For this review, take the finished solid that the model builds, in its own axes (mm). A direction names the side the tool comes from. Give positions to 0.01 mm unless a question says otherwise; leave off trailing zeros. Write each loop counter-clockwise with the first axis right and the second up, starting at its lowest first coordinate (ties: lowest second). Pieces come first, ordered by that corner, then holes.
Q1. We need section D-D (z = 2.5). Write out the cut boundary in (x, y), then the cut area to 3 significant figures.
Q2. For line 1 (Z direction, x = -2.5, y = 9.5); line 2 (Y direction, x = 0, z = 3.5); line 3 (Y direction, x = -16, z = 0.25), list the stretches that pass through material, from the lowest coordinate up.
Q3. We need section A-A (x = 16). Write out the cut boundary in (y, z) (3 decimals).
Q4. Machinability: for faces 4 (the flat face through (-7, -9, 9.5)), 5 (the cylindrical face through (-0.217, 0.976, 0.246)), 6 (the cylindrical face through (11.99, 0.53, 4.69)), which of the approach directions +Z, -Z, +X, -X, +Y, -Y give a long, thin tool a straight path to every point of the face, cutting with its end or side? Answer none if there is none.
Q5. We need section B-B (y = 0). Give the number of separate pieces and of enclosed holes in the cut face, then the cut area to 3 significant figures.
Q6. Insertion check: P1, Ø1, axis at x = -6, z = 1.5, coming from the +Y side (3 decimals); P2, Ø1.6, axis at x = -16, y = 0, coming from the +Z side; P3, Ø2.5, axis at x = 16, y = 0, coming from the +Z side; P4, Ø1.5, axis at x = -11, z = 7.5, coming from the +Y side. Each pin has a flat end and moves straight along its axis. Give the tip position at first contact, or say it passes through.
Q7. Mouldability with a two-part tool opening along X and no side actions: class faces 1 (the flat face through (-2, 0, 10)), 2 (the cylindrical face through (20, 0.1, 0.2)), 3 (the flat face through (-2, 0, 9)) as released by +X, released by -X, zero draft, split by the parting line, or undercut.
Q8. We need section C-C (x = 0). Write out the cut boundary in (y, z), then the cut area to 3 significant figures.
```python
from build123d import *

# Parameters (mm, degrees)
BOSS_EXTRU_1_DEPTH         = 0.5
ESQUISSE2_R                = 12.5
BOSS_EXTRU_2_DEPTH         = 9
ESQUISSE4_R                = 1
ENL_V_MAT_EXTRU_1_DEPTH    = 26.617376915
TROU_TARAUD_M21_AT_2_COUNT = 2
TROU_TARAUD_M21_AT_2_PITCH = 32
ESQUISSE7_R                = 12
ENL_V_MAT_EXTRU_2_DEPTH    = 9
ESQUISSE8_R                = 12
ESQUISSE8_R_2              = 1
BOSS_EXTRU_3_DEPTH         = 0.5


with BuildPart() as part:
    # Esquisse1 → Boss.-Extru.1 (new body)
    with BuildSketch(Plane.XY):
        with BuildLine():
            Line((-18.125, 3.388860428), (-6.640625, 10.590188837))
            ThreePointArc((-6.640625, 10.590188837), (0, 12.5), (6.640625, 10.590188837))
            Line((6.640625, 10.590188837), (18.125, 3.388860428))
            ThreePointArc((18.125, 3.388860428), (20, 0), (18.125, -3.388860428))
            Line((18.125, -3.388860428), (6.640625, -10.590188837))
            ThreePointArc((6.640625, -10.590188837), (0, -12.5), (-6.640625, -10.590188837))
            Line((-6.640625, -10.590188837), (-18.125, -3.388860428))
            ThreePointArc((-18.125, -3.388860428), (-20, 0), (-18.125, 3.388860428))
        make_face()
    extrude(amount=BOSS_EXTRU_1_DEPTH)

    # Esquisse2 → Boss.-Extru.2 (add)
    with BuildSketch(Plane.XY.offset(0.5)):
        with Locations(Location((0, 0, 0), (0, 0, 122.089951256))):
            Circle(ESQUISSE2_R)
    extrude(amount=BOSS_EXTRU_2_DEPTH)

    # Esquisse3 → Révolution1 (revolve)
    with BuildSketch(Plane(origin=(0, 0, 0), x_dir=(0, 0, -1), z_dir=(1, 0, 0)), mode=Mode.PRIVATE) as r_volution1_sk:
        Polygon((-9.5, 10.866025404), (-10, 10), (-10, 0), (-9.5, 0), align=None)
    revolve(r_volution1_sk.sketch.rotate(Axis((0, 0, 2.055193474), (0, 0, 1)), 90), axis=Axis((0, 0, 2.055193474), (0, 0, 1)))

    # Esquisse4 → Enlèv. mat.-Extru.1 (cut, through all)
    with BuildSketch(Plane.XY.offset(10)):
        Circle(ESQUISSE4_R)
    extrude(amount=-ENL_V_MAT_EXTRU_1_DEPTH, mode=Mode.SUBTRACT)

    # Esquisse6 → Trou taraudé M21 (revolve, cut)
    with BuildSketch(Plane(origin=(16, 0, 0.5), x_dir=(0, -1, 0), z_dir=(1, 0, 0))):
        Polygon((0, 0), (0, 6.480688495), (0.8, 6), (0.8, 4), (1, 4), (1, 0.025), (1.025, 0), align=None)
    trou_taraud_m21 = revolve(axis=Axis((16, 0, 6.85), (0, 0, -1)), mode=Mode.SUBTRACT)

    # Trou taraudé M21 at 2: Trou taraudé M21 ×2
    with Locations(*[(-i * TROU_TARAUD_M21_AT_2_PITCH, 0, 0) for i in range(1, TROU_TARAUD_M21_AT_2_COUNT)]):
        add(trou_taraud_m21, mode=Mode.SUBTRACT)

    # Esquisse7 → Enlèv. mat.-Extru.2 (cut)
    with BuildSketch(Plane(origin=(0, 0, 0), x_dir=(-1, 0, 0), z_dir=(0, 0, -1))):
        Circle(ESQUISSE7_R)
    extrude(amount=-ENL_V_MAT_EXTRU_2_DEPTH, mode=Mode.SUBTRACT)

    # Esquisse8 → Boss.-Extru.3 (add)
    with BuildSketch(Plane(origin=(0, 0, 0), x_dir=(-1, 0, 0), z_dir=(0, 0, -1))):
        Circle(ESQUISSE8_R)
        with Locations(Location((0, 0, 0), (0, 0, 180))):
            Circle(ESQUISSE8_R_2, mode=Mode.SUBTRACT)
    extrude(amount=-BOSS_EXTRU_3_DEPTH)


solid = part.part
```
Computed:
1. outline: circle Ø25 at (0, 0); hole circle Ø24 at (0, 0)
1. area: 38.5 mm2
2. line 1: z = 0 to 0.5, 9 to 10
2. line 2: y = -12.5 to -12, 12 to 12.5
2. line 3: y = -4.72 to -1, 1 to 4.72
3. outline: (-4.721, 0) - (-1, 0) - (-1, 0.475) - (-1.025, 0.5) - (-4.721, 0.5) - close; (1, 0) - (4.721, 0) - (4.721, 0.5) - (1.025, 0.5) - (1, 0.475) - close
4. face 4: +Z
4. face 5: +Z, -Z
4. face 6: none
5. separate pieces: 4
5. enclosed holes: 0
5. area: 46.4 mm2
6. P1: stops at y = 11.225
6. P2: passes through
6. P3: stops at z = 0.5
6. P4: stops at y = 7.15
7. face 1: zero draft
7. face 2: released by +X
7. face 3: undercut
8. outline: (-12.5, 0) - (-1, 0) - (-1, 0.5) - (-12, 0.5) - (-12, 9) - (-1, 9) - (-1, 10) - (-10, 10) - (-10.87, 9.5) - (-12.5, 9.5) - close; (1, 0) - (12.5, 0) - (12.5, 9.5) - (10.87, 9.5) - (10, 10) - (1, 10) - (1, 9) - (12, 9) - (12, 0.5) - (1, 0.5) - close
8. area: 40.9 mm2
